Build history of the part. All positions in model axes, mm. Give positions to 0.01 mm unless a question says otherwise; leave off trailing zeros. Write each loop counter-clockwise with the first axis right and the second up, starting at its lowest first coordinate (ties: lowest second). Pieces come first, ordered by that corner, then holes. Notation, with made-up numbers: (18.5, 16.25) -> (43.5, 16.25) arc R21 ccw to (43.5, 46.25) -> close; hole circle Ø4 at (-21, -17.5). An arc over 180 degrees is marked (long way). One line per question, with ' | ' between items. Start each with the question number.
(1) Drill centre lines: probe 1 along X at (y, z) = (-2.2, 86); probe 2 along X at (y, z) = (-2.55, 1.5); probe 3 along Z at (x, y) = (78, -2.3). Where is each one in solid material? Low to high. Write a range as from..to.
(2) Pin check, flat tips, straight feed: P1, Ø1.5, axis at x = 154.5, y = -3.5, coming from the -Z side; P2, Ø1.5, axis at y = -3, z = 108, coming from the -X side. Stop position of each tip, or through.
(3) Band-saw the part on A-A, the plane z = 47. Give the cut face in (x, y).
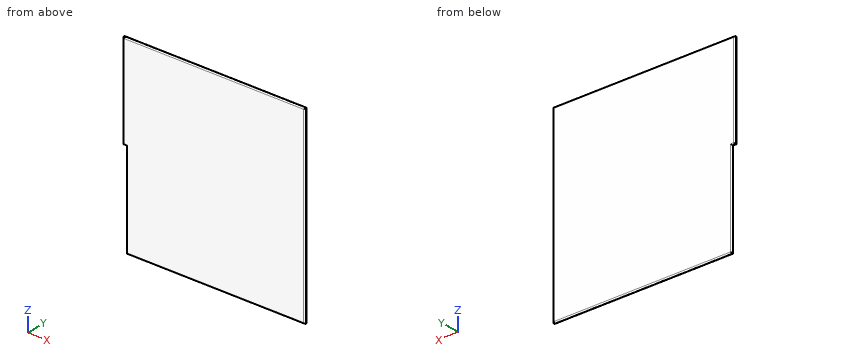
from build123d import *

# Parameters (mm, degrees)
F1_DEPTH     = 4
F2_R         = 1
F3_DEPTH     = 310
F4_T1_DEPTH  = 300
F4_T3_DEPTH  = 160
F4_T5_DEPTH  = 10
F4_T7_DEPTH  = 155
F4_T9_DEPTH  = 295
F4_T11_DEPTH = 310
F4_T17_DEPTH = 15
F4_T21_DEPTH = 160
F5_T1_DEPTH  = 300
F5_T3_DEPTH  = 160
F5_T5_DEPTH  = 10
F5_T7_DEPTH  = 155
F5_T9_DEPTH  = 295
F5_T11_DEPTH = 310
F5_T17_DEPTH = 15
F5_T21_DEPTH = 160


# Not quite as in the source:
# - a fillet or chamfer that OpenCascade refuses, or shapes differently, is made with other operations: its cross-section is extruded or revolved along the edge and cut away or added


with BuildPart() as f1:
    # F0 (on Front) → F1 (new body)
    with BuildSketch(Plane.XZ):
        Polygon((251.4121359825, 250.8489221025), (-38.5878640175, 250.8489221025), (-38.5878640175, 100.8489221025), (-33.5878640175, 100.8489221025), (-33.5878640175, -49.1510778975), (251.4121359825, -49.1510778975), align=None)
    extrude(amount=F1_DEPTH)

    # F2 (on face) → F3 (cut)
    with BuildSketch(Plane.XY.offset(250.8489221025)):
        with Locations((-36.5878640175, -2)):
            Circle(F2_R)
    extrude(amount=-F3_DEPTH, mode=Mode.SUBTRACT)

    # F4: fillet of radius 2 on 6 edges, made by hand

    # F4_s2 → F4_t1 (cut)
    with BuildSketch(Plane.YZ.offset(-43.5878640175)):
        with BuildLine():
            ThreePointArc((-2, 250.8489221025), (-3.4142135624, 250.2631356648), (-4, 248.8489221025))
            Line((-4, 248.8489221025), (-4, 250.8489221025))
            Line((-4, 250.8489221025), (-2, 250.8489221025))
        make_face()
    extrude(amount=F4_T1_DEPTH, mode=Mode.SUBTRACT)

    # F4_s4 → F4_t3 (cut)
    with BuildSketch(Plane.XY.offset(95.8489221025)):
        with BuildLine():
            ThreePointArc((-36.5878640175, -4), (-38.0020775799, -3.4142135624), (-38.5878640175, -2))
            Line((-38.5878640175, -2), (-38.5878640175, -4))
            Line((-38.5878640175, -4), (-36.5878640175, -4))
        make_face()
    extrude(amount=F4_T3_DEPTH, mode=Mode.SUBTRACT)

    # F4_s6 → F4_t5 (cut)
    with BuildSketch(Plane.YZ.offset(-43.5878640175)):
        with BuildLine():
            ThreePointArc((-4, 102.8489221025), (-3.4142135624, 101.4347085401), (-2, 100.8489221025))
            Line((-2, 100.8489221025), (-4, 100.8489221025))
            Line((-4, 100.8489221025), (-4, 102.8489221025))
        make_face()
    extrude(amount=F4_T5_DEPTH, mode=Mode.SUBTRACT)

    # F4_s8 → F4_t7 (cut)
    with BuildSketch(Plane.XY.offset(-54.1510778975)):
        with BuildLine():
            ThreePointArc((-31.5878640175, -4), (-33.0020775799, -3.4142135624), (-33.5878640175, -2))
            Line((-33.5878640175, -2), (-33.5878640175, -4))
            Line((-33.5878640175, -4), (-31.5878640175, -4))
        make_face()
    extrude(amount=F4_T7_DEPTH, mode=Mode.SUBTRACT)

    # F4_s10 → F4_t9 (cut)
    with BuildSketch(Plane.YZ.offset(-38.5878640175)):
        with BuildLine():
            ThreePointArc((-4, -47.1510778975), (-3.4142135624, -48.5652914599), (-2, -49.1510778975))
            Line((-2, -49.1510778975), (-4, -49.1510778975))
            Line((-4, -49.1510778975), (-4, -47.1510778975))
        make_face()
    extrude(amount=F4_T9_DEPTH, mode=Mode.SUBTRACT)

    # F4_s12 → F4_t11 (cut)
    with BuildSketch(Plane.XY.offset(-54.1510778975)):
        with BuildLine():
            ThreePointArc((251.4121359825, -2), (250.8263495449, -3.4142135624), (249.4121359825, -4))
            Line((249.4121359825, -4), (251.4121359825, -4))
            Line((251.4121359825, -4), (251.4121359825, -2))
        make_face()
    extrude(amount=F4_T11_DEPTH, mode=Mode.SUBTRACT)


with BuildPart() as f4_tool15:
    # F4_s16 → F4_t17 (new body)
    with BuildSketch(Plane.YZ.offset(-43.5878640175)):
        with BuildLine():
            ThreePointArc((-4, 102.8489221025), (-3.4142135624, 101.4347085401), (-2, 100.8489221025))
            Line((-2, 100.8489221025), (-4, 100.8489221025))
            Line((-4, 100.8489221025), (-4, 102.8489221025))
        make_face()
    extrude(amount=F4_T17_DEPTH)

    split(bisect_by=Plane.YZ.offset(-33.5878640175), keep=Keep.TOP)


with BuildPart() as f4_tool19:
    # F4_s20 → F4_t21 (new body)
    with BuildSketch(Plane.XY.offset(105.8489221025)):
        with BuildLine():
            ThreePointArc((-31.5878640175, -4), (-33.0020775799, -3.4142135624), (-33.5878640175, -2))
            Line((-33.5878640175, -2), (-33.5878640175, -4))
            Line((-33.5878640175, -4), (-31.5878640175, -4))
        make_face()
    extrude(amount=-F4_T21_DEPTH)

    split(bisect_by=Plane.XY.offset(100.8489221025), keep=Keep.TOP)


with BuildPart() as f4_tool15_1:
    add(f4_tool15.part)

    # F4_t23: intersect F4_tool19
    add(f4_tool19.part, mode=Mode.INTERSECT)


with BuildPart() as f1_1:
    add(f1.part)

    # F4_t13: cut F4_tool15
    add(f4_tool15_1.part, mode=Mode.SUBTRACT)

    # F5: fillet of radius 2 on 6 edges, made by hand

    # F5_s2 → F5_t1 (cut)
    with BuildSketch(Plane.YZ.offset(-43.5878640175)):
        with BuildLine():
            ThreePointArc((-2, 250.8489221025), (-0.5857864376, 250.2631356648), (0, 248.8489221025))
            Line((0, 248.8489221025), (0, 250.8489221025))
            Line((0, 250.8489221025), (-2, 250.8489221025))
        make_face()
    extrude(amount=F5_T1_DEPTH, mode=Mode.SUBTRACT)

    # F5_s4 → F5_t3 (cut)
    with BuildSketch(Plane.XY.offset(95.8489221025)):
        with BuildLine():
            ThreePointArc((-36.5878640175, 0), (-38.0020775799, -0.5857864376), (-38.5878640175, -2))
            Line((-38.5878640175, -2), (-38.5878640175, 0))
            Line((-38.5878640175, 0), (-36.5878640175, 0))
        make_face()
    extrude(amount=F5_T3_DEPTH, mode=Mode.SUBTRACT)

    # F5_s6 → F5_t5 (cut)
    with BuildSketch(Plane.YZ.offset(-43.5878640175)):
        with BuildLine():
            ThreePointArc((0, 102.8489221025), (-0.5857864376, 101.4347085401), (-2, 100.8489221025))
            Line((-2, 100.8489221025), (0, 100.8489221025))
            Line((0, 100.8489221025), (0, 102.8489221025))
        make_face()
    extrude(amount=F5_T5_DEPTH, mode=Mode.SUBTRACT)

    # F5_s8 → F5_t7 (cut)
    with BuildSketch(Plane.XY.offset(-54.1510778975)):
        with BuildLine():
            ThreePointArc((-31.5878640175, 0), (-33.0020775799, -0.5857864376), (-33.5878640175, -2))
            Line((-33.5878640175, -2), (-33.5878640175, 0))
            Line((-33.5878640175, 0), (-31.5878640175, 0))
        make_face()
    extrude(amount=F5_T7_DEPTH, mode=Mode.SUBTRACT)

    # F5_s10 → F5_t9 (cut)
    with BuildSketch(Plane.YZ.offset(-38.5878640175)):
        with BuildLine():
            ThreePointArc((0, -47.1510778975), (-0.5857864376, -48.5652914599), (-2, -49.1510778975))
            Line((-2, -49.1510778975), (0, -49.1510778975))
            Line((0, -49.1510778975), (0, -47.1510778975))
        make_face()
    extrude(amount=F5_T9_DEPTH, mode=Mode.SUBTRACT)

    # F5_s12 → F5_t11 (cut)
    with BuildSketch(Plane.XY.offset(-54.1510778975)):
        with BuildLine():
            ThreePointArc((249.4121359825, 0), (250.8263495449, -0.5857864376), (251.4121359825, -2))
            Line((251.4121359825, -2), (251.4121359825, 0))
            Line((251.4121359825, 0), (249.4121359825, 0))
        make_face()
    extrude(amount=F5_T11_DEPTH, mode=Mode.SUBTRACT)


with BuildPart() as f5_tool15:
    # F5_s16 → F5_t17 (new body)
    with BuildSketch(Plane.YZ.offset(-43.5878640175)):
        with BuildLine():
            ThreePointArc((0, 102.8489221025), (-0.5857864376, 101.4347085401), (-2, 100.8489221025))
            Line((-2, 100.8489221025), (0, 100.8489221025))
            Line((0, 100.8489221025), (0, 102.8489221025))
        make_face()
    extrude(amount=F5_T17_DEPTH)

    split(bisect_by=Plane.YZ.offset(-33.5878640175), keep=Keep.TOP)


with BuildPart() as f5_tool19:
    # F5_s20 → F5_t21 (new body)
    with BuildSketch(Plane.XY.offset(105.8489221025)):
        with BuildLine():
            ThreePointArc((-31.5878640175, 0), (-33.0020775799, -0.5857864376), (-33.5878640175, -2))
            Line((-33.5878640175, -2), (-33.5878640175, 0))
            Line((-33.5878640175, 0), (-31.5878640175, 0))
        make_face()
    extrude(amount=-F5_T21_DEPTH)

    split(bisect_by=Plane.XY.offset(100.8489221025), keep=Keep.TOP)


with BuildPart() as f5_tool15_1:
    add(f5_tool15.part)

    # F5_t23: intersect F5_tool19
    add(f5_tool19.part, mode=Mode.INTERSECT)


with BuildPart() as f1_2:
    add(f1_1.part)

    # F5_t13: cut F5_tool15
    add(f5_tool15_1.part, mode=Mode.SUBTRACT)


solid = f1_2.part
Results:
1) probe 1: x = -33.58..251.4 | probe 2: x = -33.51..251.34 | probe 3: z = -49.13..250.83
2) P1: stops at z = -49.01 | P2: stops at x = -38.57
3) outline: (-31.59, -4) -> (249.41, -4) arc R2 ccw to (249.41, 0) -> (-31.59, 0) arc R2 ccw to start
